Could you check a few things on this model? Use its own coordinates, in mm. A direction names the side the tool comes from. Coordinates: 2 decimals unless noted, no trailing zeros. Loops run counter-clockwise (first coordinate to the right, second up) from the corner with the lowest first, then second, coordinate; pieces in that order, holes last.
from build123d import *

# Parameters (mm, degrees)
F1_DEPTH = 8.89


with BuildPart() as f1:
    # F0 (on Top) → F1 (new body)
    with BuildSketch(Plane.XY):
        Polygon((19.05, 0), (8.89, 0), (8.89, -19.05), (0, -19.05), (0, -31.75), (8.89, -31.75), (8.89, -44.45), (0, -44.45), (0, -57.15), (8.89, -57.15), (8.89, -69.85), (0, -69.85), (0, -82.55), (8.89, -82.55), (8.89, -95.25), (0, -95.25), (0, -107.95), (8.89, -107.95), (8.89, -120.65), (0, -120.65), (0, -133.35), (8.89, -133.35), (8.89, -146.05), (0, -146.05), (0, -158.75), (8.89, -158.75), (8.89, -177.8), (19.05, -177.8), (19.05, -168.91), (31.75, -168.91), (31.75, -177.8), (44.45, -177.8), (44.45, -168.91), (57.15, -168.91), (57.15, -177.8), (69.85, -177.8), (69.85, -168.91), (82.55, -168.91), (82.55, -177.8), (95.25, -177.8), (95.25, -168.91), (107.95, -168.91), (107.95, -177.8), (120.65, -177.8), (120.65, -168.91), (133.35, -168.91), (133.35, -177.8), (146.05, -177.8), (146.05, -168.91), (158.75, -168.91), (158.75, -177.8), (168.91, -177.8), (168.91, -158.75), (177.8, -158.75), (177.8, -146.05), (168.91, -146.05), (168.91, -133.35), (177.8, -133.35), (177.8, -120.65), (168.91, -120.65), (168.91, -107.95), (177.8, -107.95), (177.8, -95.25), (168.91, -95.25), (168.91, -82.55), (177.8, -82.55), (177.8, -69.85), (168.91, -69.85), (168.91, -57.15), (177.8, -57.15), (177.8, -44.45), (168.91, -44.45), (168.91, -31.75), (177.8, -31.75), (177.8, -19.05), (168.91, -19.05), (168.91, 0), (158.75, 0), (158.75, -8.89), (146.05, -8.89), (146.05, 0), (133.35, 0), (133.35, -8.89), (120.65, -8.89), (120.65, 0), (107.95, 0), (107.95, -8.89), (95.25, -8.89), (95.25, 0), (82.55, 0), (82.55, -8.89), (69.85, -8.89), (69.85, 0), (57.15, 0), (57.15, -8.89), (44.45, -8.89), (44.45, 0), (31.75, 0), (31.75, -8.89), (19.05, -8.89), align=None)
        with BuildLine():
            ThreePointArc((31.75, -71.12), (33.609872, -66.629872), (38.1, -64.77))
            Line((38.1, -64.77), (139.7, -64.77))
            ThreePointArc((139.7, -64.77), (144.190128, -66.629872), (146.05, -71.12))
            Line((146.05, -71.12), (146.05, -81.915))
            ThreePointArc((146.05, -81.915), (144.190128, -86.405128), (139.7, -88.265))
            Line((139.7, -88.265), (38.1, -88.265))
            ThreePointArc((38.1, -88.265), (33.609872, -86.405128), (31.75, -81.915))
            Line((31.75, -81.915), (31.75, -71.12))
        make_face(mode=Mode.SUBTRACT)
    extrude(amount=F1_DEPTH)


solid = f1.part
(1) Which directions (+Z, -Z, +X, -X, +Y, -Y) give clear straight access to the entire face, cutting with the end or side of a thin tool? Please do faces 1 (the face through (144.14, -66.58, 4.38)), 2 (the face through (173, -19.05, 4)), 3 (the face through (146.05, -173, 4)), 4 (the face through (173, -95.25, 4)).
Answers:
face 1: +Z, -Z
face 2: +Z, -Z, +X, +Y
face 3: +Z, -Z, -Y
face 4: +Z, -Z, +X
(2) For pin 1 (4.5 mm diameter, centred on y = -166, z = 4.5, fed in from -X); pin 2 (4.5 mm diameter, centred on x = 79, z = 3, fed in from -Y); pin 3 (2.5 mm diameter, centred on x = 129, z = 5.5, fed in from +Y), each with a flat end and sliding along its axis, tell me the tip position at first contact or that it passes through.
Answers:
pin 1: stops at x = 8.89
pin 2: stops at y = -168.91
pin 3: stops at y = -8.89
(3) I need wall thicknesses on probe 1 along Y at (x, z) = (171.5, 5.75); probe 2 along Y at (x, z) = (102, 1) (3 decimals); probe 3 along Y at (x, z) = (67, 7.5) (3 decimals). Which ranges of each line are inside material? Lowest first, please.
Answers:
probe 1: y = -158.75 to -146.05, -133.35 to -120.65, -107.95 to -95.25, -82.55 to -69.85, -57.15 to -44.45, -31.75 to -19.05
probe 2: y = -168.91 to -88.265, -64.77 to -8.89
probe 3: y = -177.8 to -88.265, -64.77 to 0
(4) We'd pull the mould along X, two halves only. Please class faces 5 (the face through (31.75, -4, 4)), 6 (the face through (5, -120.65, 4)), 7 (the face through (8.89, -9, 4)): +X half, -X half, draft (parallel to the pull), parting line (faces both ways), or undercut.
Answers:
face 5: undercut
face 6: draft
face 7: -X half
(5) Imagine slicing it at A-A, the plane x = 75.5. Write out the boundary of the cut face in (y, z) (3 decimals), and give its area (3 significant figures).
Answers:
outline: (-168.91, 0) - (-88.265, 0) - (-88.265, 8.89) - (-168.91, 8.89) - close; (-64.77, 0) - (-8.89, 0) - (-8.89, 8.89) - (-64.77, 8.89) - close
area: 1,210 mm2
(6) Imagine slicing it at B-B, the plane y = -67.5. Write out the boundary of the cut face in (x, z), and give its area (3 significant figures).
Answers:
outline: (8.89, 0) - (32.88, 0) - (32.88, 8.89) - (8.89, 8.89) - close; (144.92, 0) - (168.91, 0) - (168.91, 8.89) - (144.92, 8.89) - close
area: 427 mm2
(7) Imagine slicing it at C-C, the plane y = -162. Write out the boundary of the cut face in (x, z).
Answers:
outline: (8.89, 0) - (168.91, 0) - (168.91, 8.89) - (8.89, 8.89) - close
